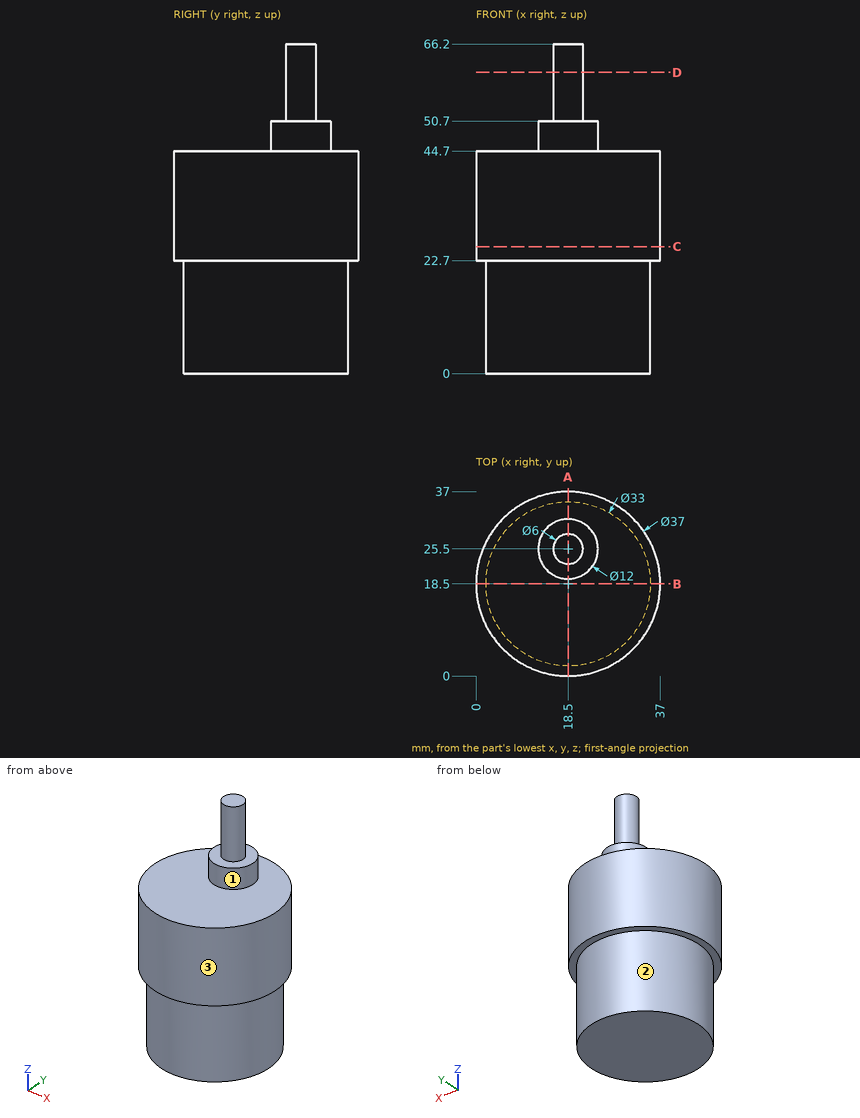
Could you check a few things on this drawing? It's one solid part, dimensions in mm from its lowest x, y, z. A direction names the side the tool comes from. Round coordinates to 2 decimals unless told otherwise and drop trailing zeros. Order: outer loops, then holes, each group sorted by start corner. A loop starts at its lowest first (then second) coordinate and runs counter-clockwise, first axis right, second up. Notation, with made-up numbers: M 25,89 L 64,89 A24 ccw 64,110 Z; hole C -38.5,79.25 d7. An arc over 180 degrees is marked long. Return JSON: item names as keys, results as strings. Group by question number.
1. If we section it at C-C on z = 25.5: List the corners of the cut face in (x, y) for me.
2. If we section it at A-A on x = 18.5: List the corners of the cut face in (y, z) for me, then the cut area to 3 significant figures.
3. If we section it at B-B on y = 18.5: List the corners of the cut face in (x, z) for me.
4. I'm going to push flat-ended pins straight in: pin 1 Ø2 at (y, z) = (25, 40.5) entering from -X; pin 2 Ø2 at (y, z) = (12.5, 35.5) entering from +X; pin 3 Ø1 at (y, z) = (32.5, 22.5) entering from +X. Where does each tip first touch, or does it pass through?
5. On a 3-axis mill with a long thin cutter (end or side, diameter ignored), from which of +Z, -Z, +X, -X, +Y, -Y can I reach the whole of each face in a straight line? I mean the marked faces 1, 2 and 3. Say none if no direction works.
6. Please list where these lines run through material, in increasing order: probe 1 along Z at (x, y) = (5.5, 19.5); probe 2 along Y at (x, z) = (4, 24.5); probe 3 along X at (y, z) = (28.5, 17.5).
7. If we section it at D-D on z = 60.5: List the corners of the cut face in (x, y) for me.
Reply:
{
 "1": {"outline": "C 18.5,18.5 d37"},
 "2": {"outline": "M 0,22.7 L 2,22.7 L 2,0 L 35,0 L 35,22.7 L 37,22.7 L 37,44.7 L 31.5,44.7 L 31.5,50.7 L 28.5,50.7 L 28.5,66.2 L 22.5,66.2 L 22.5,50.7 L 19.5,50.7 L 19.5,44.7 L 0,44.7 Z", "area": "1,730 mm^2"},
 "3": {"outline": "M 0,22.7 L 2,22.7 L 2,0 L 35,0 L 35,22.7 L 37,22.7 L 37,44.7 L 0,44.7 Z"},
 "4": {"pin 1": "x = 0.84", "pin 2": "x = 36.31", "pin 3": "x = 31.1"},
 "5": {"face 1": "+Z", "face 2": "-Z", "face 3": "+Z, -Z"},
 "6": {"probe 1": "0 to 44.7", "probe 2": "7.01 to 29.99", "probe 3": "5.38 to 31.62"},
 "7": {"outline": "C 18.5,25.5 d6"}
}
